Verification items for the finished model (mm, model axes). A direction names the side the tool comes from. Round coordinates to 2 decimals unless told otherwise and drop trailing zeros. Loops run counter-clockwise (first coordinate to the right, second up) from the corner with the lowest first, then second, coordinate; pieces in that order, holes last. Notation, with made-up numbers: (-14, 15.25) - (-2, 15.25) arc R28 cw to (-2, 50.25) - close; hole circle Ø1 at (-32.5, -10.75). An arc over 180 degrees is marked (long way). Use a Markdown table: item, result. Add a question column.
```python
from build123d import *

# Parameters (mm, degrees)
SKETCH1_W                 = 50.8
SKETCH1_H                 = 25.4
SKETCH1_W_2               = 44.45
SKETCH1_H_2               = 19.05
BOSS_EXTRUDE1_DEPTH       = 244.7925
SKETCH2_W                 = 25.4
SKETCH2_H                 = 50.8
CUT_EXTRUDE1_DEPTH        = 248.414001334
SKETCH3_W                 = 25.4
SKETCH3_H                 = 63.5
CUT_EXTRUDE2_DEPTH        = 248.414001334
F_8_32_TAPPED_HOLE1_D     = 3.4544
F_8_32_TAPPED_HOLE2_D     = 3.4544
CUT_EXTRUDE3_DEPTH        = 248.414001334
FILLET1_R                 = 4.7625
F_8_32_TAPPED_HOLE3_D     = 3.4544
F_8_32_TAPPED_HOLE4_D     = 3.4544
F_8_32_TAPPED_HOLE4_DEPTH = 3.175
F_8_32_TAPPED_HOLE5_D     = 3.4544


with BuildPart() as part:
    # Sketch1 → Boss-Extrude1 (new, symmetric)
    with BuildSketch(Plane(origin=(0, 0, 0), x_dir=(1, 0, 0), z_dir=(0, 1, 0))):
        Rectangle(SKETCH1_W, SKETCH1_H)
        Rectangle(SKETCH1_W_2, SKETCH1_H_2, mode=Mode.SUBTRACT)
    extrude(amount=BOSS_EXTRUDE1_DEPTH, both=True)

    # Sketch2 → Cut-Extrude1 (cut, through all)
    with BuildSketch(Plane.XY.offset(12.7)):
        with Locations((12.7, 219.3925)):
            Rectangle(SKETCH2_W, SKETCH2_H)
    extrude(amount=-CUT_EXTRUDE1_DEPTH, mode=Mode.SUBTRACT)

    # Sketch3 → Cut-Extrude2 (cut, through all)
    with BuildSketch(Plane.XY.offset(12.7)):
        with Locations((-12.7, -12.3825)):
            Rectangle(SKETCH3_W, SKETCH3_H)
    extrude(amount=-CUT_EXTRUDE2_DEPTH, mode=Mode.SUBTRACT)

    # #8-32 Tapped Hole1 (through all)
    with Locations(Plane(origin=(0, 0, -12.7), x_dir=(-1, 0, 0), z_dir=(0, 0, -1))):
        with Locations((12.7, 232.0925), (12.7, 206.6925), (12.7, 181.2925), (-12.7, 181.2925)):
            Hole(F_8_32_TAPPED_HOLE1_D / 2)

    # #8-32 Tapped Hole2 (through all)
    with Locations(Plane.XY.offset(12.7)):
        with Locations((-15.875, 238.4425), (-15.875, 200.3425)):
            Hole(F_8_32_TAPPED_HOLE2_D / 2)

    # Sketch8 → Cut-Extrude3 (cut, through all)
    with BuildSketch(Plane.XY.offset(12.7)):
        Polygon((15.875, -219.3925), (15.875, -179.453847181), (-15.875, -219.3925), align=None)
        Polygon((-15.875, -204.086152819), (15.875, -164.1475), (-15.875, -124.208847181), align=None)
        Polygon((-15.875, -108.9025), (15.875, -148.841152819), (15.875, -68.963847181), align=None)
        Polygon((-15.875, -93.596152819), (15.875, -53.6575), (-15.875, -53.6575), align=None)
        Polygon((-15.875, 28.8925), (15.875, 28.8925), (15.875, 61.751507535), align=None)
        Polygon((-15.875, 42.600159131), (15.875, 75.459166667), (-15.875, 108.318174202), align=None)
        Polygon((-15.875, 122.025833333), (15.875, 89.166825798), (15.875, 154.884840869), align=None)
        Polygon((-15.875, 168.5925), (-15.875, 135.733492465), (15.875, 168.5925), align=None)
    extrude(amount=-CUT_EXTRUDE3_DEPTH, mode=Mode.SUBTRACT)

    # Fillet1
    fillet1_edges = [part.edges().sort_by_distance(p)[0] for p in [
        (-15.875, -204.086152819, -11.1125),
        (-15.875, -124.208847181, -11.1125),
        (15.875, -164.1475, -11.1125),
        (-15.875, -204.086152819, 11.1125),
        (-15.875, -124.208847181, 11.1125),
        (15.875, -164.1475, 11.1125),
        (15.875, -148.841152819, -11.1125),
        (-15.875, -108.9025, -11.1125),
        (15.875, -68.963847181, -11.1125),
        (15.875, -148.841152819, 11.1125),
        (-15.875, -108.9025, 11.1125),
        (15.875, -68.963847181, 11.1125),
        (-15.875, -93.596152819, -11.1125),
        (-15.875, -53.6575, -11.1125),
        (15.875, -53.6575, -11.1125),
        (-15.875, -93.596152819, 11.1125),
        (-15.875, -53.6575, 11.1125),
        (15.875, -53.6575, 11.1125),
        (15.875, 61.751507535, -11.1125),
        (15.875, 28.8925, -11.1125),
        (-15.875, 28.8925, -11.1125),
        (15.875, 61.751507535, 11.1125),
        (15.875, 28.8925, 11.1125),
        (-15.875, 28.8925, 11.1125),
        (-15.875, 42.600159131, -11.1125),
        (-15.875, 108.318174202, -11.1125),
        (15.875, 75.459166667, -11.1125),
        (-15.875, 42.600159131, 11.1125),
        (-15.875, 108.318174202, 11.1125),
        (15.875, 75.459166667, 11.1125),
        (15.875, 89.166825798, -11.1125),
        (-15.875, 122.025833333, -11.1125),
        (15.875, 154.884840869, -11.1125),
        (15.875, 89.166825798, 11.1125),
        (-15.875, 122.025833333, 11.1125),
        (15.875, 154.884840869, 11.1125),
        (-15.875, 135.733492465, -11.1125),
        (-15.875, 168.5925, -11.1125),
        (15.875, 168.5925, -11.1125),
        (-15.875, 135.733492465, 11.1125),
        (-15.875, 168.5925, 11.1125),
        (15.875, 168.5925, 11.1125),
        (-15.875, -219.3925, -11.1125),
        (15.875, -179.453847181, -11.1125),
        (15.875, -219.3925, -11.1125),
        (-15.875, -219.3925, 11.1125),
        (15.875, -179.453847181, 11.1125),
        (15.875, -219.3925, 11.1125),
    ]]
    fillet(fillet1_edges, radius=FILLET1_R)

    # #8-32 Tapped Hole3 (through all)
    with Locations(Plane.XY.offset(12.7)):
        with Locations((12.7, 3.4925)):
            Hole(F_8_32_TAPPED_HOLE3_D / 2)

    # #8-32 Tapped Hole4
    with Locations(Plane.ZY.offset(25.4)):
        with Locations((0, 32.0675), (0, 57.4675), (0, -56.8325), (0, -82.2325)):
            Hole(F_8_32_TAPPED_HOLE4_D / 2, depth=F_8_32_TAPPED_HOLE4_DEPTH)

    # #8-32 Tapped Hole5 (through all)
    with Locations(Plane.XY.offset(12.7)):
        with Locations((-19.05, -228.9175), (19.05, -228.9175)):
            Hole(F_8_32_TAPPED_HOLE5_D / 2)


solid = part.part
```
Q1. Thickness scan on line 1 along X through (y, z) = (158.5, -7.25) (3 decimals); line 2 along Z through (x, y) = (-21.5, 30) (3 decimals); line 3 along Y through (x, z) = (-22.5, 4.5). Record the ranges inside material, lowest first.
Q2. Set-up check for faces 1 (the face through (5, 3, 12.7)), 2 (the face through (5, 3, -9.525)), 3 (the face through (-2.921, -92.607, 11.135)): record each of +Z, -Z, +X, -X, +Y, -Y from which the full face is reachable in a straight line by a thin tool's end or side.
Q3. Section check A-A on y = -29. Record the cut outline in (x, z) (3 decimals).
Q4. Go/stop test with flat-tipped pins: pin 1 Ø7.5 at (x, z) = (-6.5, -4.5) entering from -Y; pin 2 Ø3 at (y, z) = (-56.83, 0) entering from -X (3 decimals); pin 3 Ø4 at (x, y) = (-19.05, -228.92) entering from -Z; pin 4 Ø3.5 at (x, z) = (2.5, 11) entering from +Y. Record where each tip stops, or that it passes through.
Q5. Release check for a two-part mould opening along X. For faces 4 (the face through (2.35, 61.46, -11.09)), 5 (the face through (5, 3, -12.7)), 6 (the face through (-25.4, -143, 0)) record: +X half, -X half, draft (parallel to the pull), parting line (faces both ways), or undercut.
Determined:
| question | item | result |
|---|---|---|
| 1 | line 1 | x = -25.4 to -22.225, 22.225 to 25.4 |
| 1 | line 2 | z = -12.7 to -9.525, 9.525 to 12.7 |
| 1 | line 3 | y = -244.79 to -44.13, 19.37 to 244.79 |
| 2 | face 1 | +Z, +X, -X, +Y, -Y |
| 2 | face 2 | +Y, -Y |
| 2 | face 3 | +Z, -Z |
| 3 | outline | (0, -12.7) - (25.4, -12.7) - (25.4, 12.7) - (0, 12.7) - (0, 9.525) - (22.225, 9.525) - (22.225, -9.525) - (0, -9.525) - close |
| 4 | pin 1 | passes through |
| 4 | pin 2 | stops at x = 22.225 |
| 4 | pin 3 | stops at z = -12.7 |
| 4 | pin 4 | stops at y = 193.99 |
| 5 | face 4 | undercut |
| 5 | face 5 | draft |
| 5 | face 6 | -X half |
